from build123d import *

# Parameters (mm, degrees)
ESQUISSE1_R             = 2.5
BOSS_EXTRU_1_DEPTH      = 40
ENL_V_MAT_EXTRU_1_DEPTH = 60
CONG_1_R                = 10
ENL_V_MAT_EXTRU_2_DEPTH = 20
ENL_V_MAT_EXTRU_3_DEPTH = 20


with BuildPart() as part:
    # Esquisse1 → Boss.-Extru.1 (new body)
    with BuildSketch(Plane(origin=(0, 0, 0), x_dir=(0, 0, -1), z_dir=(1, 0, 0))):
        with BuildLine():
            Line((0, 10), (75, 10))
            Line((75, 10), (75, 30))
            Line((75, 30), (0, 30))
            ThreePointArc((0, 30), (-48.023431781, 13.154289726), (-75, -30))
            ThreePointArc((-75, -30), (-42.5, -0.625), (0, 10))
        make_face()
        with Locations((65, 20)):
            Circle(ESQUISSE1_R, mode=Mode.SUBTRACT)
    extrude(amount=BOSS_EXTRU_1_DEPTH)

    # Esquisse2 → Enlèv. mat.-Extru.1 (cut)
    with BuildSketch(Plane(origin=(0, 30, 0), x_dir=(1, 0, 0), z_dir=(0, 1, 0))):
        Polygon((20, 0), (5, -75), (35, -75), align=None)
        Polygon((0, 75), (5, 75), (5, 0), (0, -75), align=None)
        Polygon((40, 75), (35, 75), (35, 0), (40, -75), align=None)
    extrude(amount=-ENL_V_MAT_EXTRU_1_DEPTH, mode=Mode.SUBTRACT)

    # Congé1
    cong_1_edges = [part.edges().sort_by_distance(p)[0] for p in [
        (20, 10, -75),
        (20, 30, -75),
    ]]
    fillet(cong_1_edges, radius=CONG_1_R - 0.0001)  # a hair under: the kernel refuses the full size

    # Esquisse3 → Enlèv. mat.-Extru.2 (cut)
    with BuildSketch(Plane(origin=(0, 30, 0), x_dir=(1, 0, 0), z_dir=(0, 1, 0))):
        Polygon((35, 82), (35, 55), (32, 55), (32, 80), (29, 80), (29, 55), (26, 55), (26, 80), (23, 80), (23, 55), (20, 55), (20, 80), (17, 80), (17, 55), (14, 55), (14, 80), (11, 80), (11, 55), (8, 55), (8, 82), align=None)
    extrude(amount=-ENL_V_MAT_EXTRU_2_DEPTH, mode=Mode.SUBTRACT)

    # Esquisse4 → Enlèv. mat.-Extru.3 (cut)
    with BuildSketch(Plane(origin=(0, 30, 0), x_dir=(1, 0, 0), z_dir=(0, 1, 0))):
        Polygon((8.5, 37.5), (8.5, 34.5), (16.5, 34.5), (10, 21.5), (13, 21.5), (21, 37.5), align=None)
        with BuildLine():
            Line((31, 21.5), (28, 21.5))
            Line((28, 21.5), (22.5, 27.5))
            Line((22.5, 27.5), (22.5, 30.5))
            Line((22.5, 30.5), (26.5, 30.5))
            ThreePointArc((26.5, 30.5), (28.75, 32.75), (26.5, 35))
            Line((26.5, 35), (22.5, 35))
            Line((22.5, 35), (22.5, 37.5))
            Line((22.5, 37.5), (26, 37.5))
            ThreePointArc((26, 37.5), (31.269677958, 33.000344118), (26.5, 27.973756706))
            Line((26.5, 27.973756706), (25.065723019, 27.973756706))
            Line((25.065723019, 27.973756706), (31, 21.5))
        make_face()
    extrude(amount=-ENL_V_MAT_EXTRU_3_DEPTH, mode=Mode.SUBTRACT)


solid = part.part
Build history of the part. All positions in model axes, mm. A direction names the side the tool comes from. Coordinates: 2 decimals unless noted, no trailing zeros. Write each loop counter-clockwise with the first axis right and the second up, starting at its lowest first coordinate (ties: lowest second). Pieces come first, ordered by that corner, then holes.
(1) Cut at B-B on y = -12.5. List the corners of the cut face in (x, z), and give its area (3 significant figures).
(2) 3-axis set-ups, long thin cutter, end or side, ignore diameter. For faces 4 (the flat face through (20, 10, -32)), 5 (the flat face through (12, 20, -34.5)), 6 (the flat face through (35, 20, -28)): which of +Z, -Z, +X, -X, +Y, -Y reach the whole face in a straight line?
(3) Pin check, flat tips, straight feed: pin 1 Ø6 at (y, z) = (20, -65) entering from +X; pin 2 Ø6 at (y, z) = (-6, 51) entering from -X; pin 3 Ø10 at (y, z) = (18, -40) entering from +X; pin 4 Ø2 at (x, y) = (24.5, 20.5) entering from -Z. Stop position of each tip, or through.
(4) Cut at A-A on z = -57. List the corners of the cut face in (x, y).
(5) Cut at D-D on z = -32.75. List the corners of the cut face in (x, y) (3 decimals), and give its area (3 significant figures).
(6) Cut at C-C on z = 38.5. List the corners of the cut face in (x, y).
(7) Mould opens along Z. For faces 1 (the cylindrical face through (12.48, 22.11, -66.34)), 2 (the flat face through (34, 20, -55)), 3 (the flat face through (5, 20, -38)) say: pulls with the +Z half, pulls with the -Z half, needs draft (parallel to the pull), parting line crosses it, or undercut.
(8) Drill centre lines: line 1 (X direction, y = 24, z = -57); line 2 (Y direction, x = 18, z = -65); line 3 (Z direction, x = 30, y = 20). Where is each one in solid material? Low to high.
Working result:
1. outline: (0.42, 68.76) - (1.02, 59.65) - (8.07, 59.65) - (6.25, 68.76) - close; (31.93, 59.65) - (38.98, 59.65) - (39.58, 68.76) - (33.75, 68.76) - close
1. area: 117 mm2
2. face 4: -Z, +X, -X, -Y
2. face 5: +Y, -Y
2. face 6: -Z, +X, +Y, -Y
3. pin 1: stops at x = 32
3. pin 2: stops at x = 1.4
3. pin 3: stops at x = 35
3. pin 4: stops at z = -75
4. outline: (5, 10) - (8, 10) - (8, 30) - (5, 30) - close; (11, 10) - (14, 10) - (14, 30) - (11, 30) - close; (17, 10) - (20, 10) - (20, 30) - (17, 30) - close; (23, 10) - (26, 10) - (26, 30) - (23, 30) - close; (29, 10) - (32, 10) - (32, 30) - (29, 30) - close
5. outline: (5, 10) - (15.625, 10) - (15.625, 30) - (5, 30) - close; (18.625, 10) - (28.75, 10) - (28.75, 30) - (18.625, 30) - close; (31.276, 10) - (35, 10) - (35, 30) - (31.276, 30) - close
5. area: 489 mm2
6. outline: (2.43, 1.38) - (12.3, 1.38) - (12.3, 19.66) - (2.43, 19.66) - close; (27.7, 1.38) - (37.57, 1.38) - (37.57, 19.66) - (27.7, 19.66) - close
7. face 1: undercut
7. face 2: pulls with the -Z half
7. face 3: needs draft
8. line 1: x = 5 to 8, 11 to 14, 17 to 20, 23 to 26, 29 to 32
8. line 2: y = 10 to 17.5, 22.5 to 30
8. line 3: z = -75 to -67.5, -62.5 to -36, -29.5 to -22.59, -21.5 to 37.91
